Drawing for the job (mm, zero at the part's lowest x, y, z). A direction names the side the tool comes from. Give positions to 0.01 mm unless a question says otherwise; leave off trailing zeros. Order: outer loops, then holes, each group sorted by start corner. A loop starts at its lowest first (then second) coordinate and runs counter-clockwise, first axis right, second up. Notation, with made-up numbers: M 18.5,32 L 30.5,32 A12 ccw 30.5,45 Z; hole C 83.25,76 d1. An arc over 180 degrees is marked long. Answer as a JSON object with one key per item and string values.
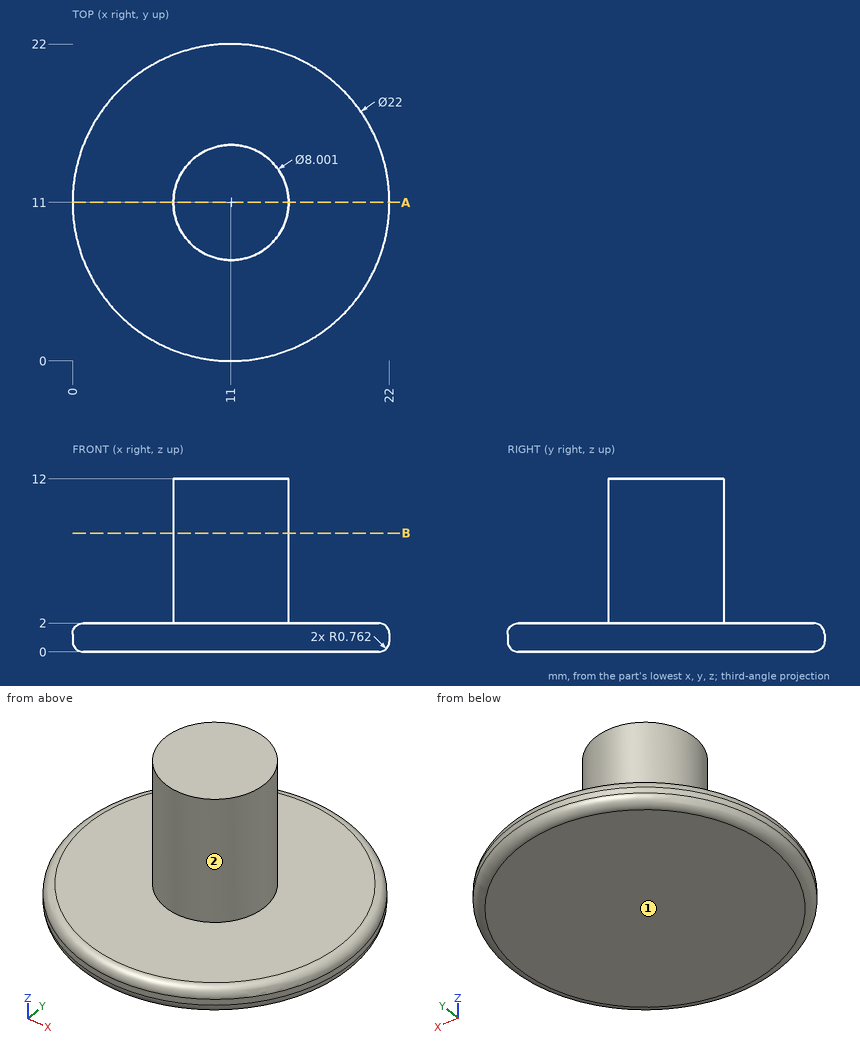
1. Cut at A-A on y = 11. Give the cut face in (x, z).
Worked answers:
{"outline": "M 0,0.76 A0.76 ccw 0.76,0 L 21.24,0 A0.76 ccw 22,0.76 L 22,1.24 A0.76 ccw 21.24,2 L 15,2 L 15,12 L 7,12 L 7,2 L 0.76,2 A0.76 ccw 0,1.24 Z"}
2. Pin check, flat tip, straight feed: P1, Ø5, axis at x = 6.5, y = 5.5, coming from the -Z side. Stop position of the tip, or through.
Worked answers:
{"P1": "stops at z = 0"}
3. Probe line 1 along Z through (x, y) = (18.5, 8); line 2 along Y through (x, z) = (17.25, 1.5); line 3 along Y through (x, z) = (20.25, 1.75). List the from-to ranges inside material, lowest first.
Worked answers:
{"line 1": "z = 0 to 2", "line 2": "y = 2 to 20", "line 3": "y = 5.42 to 16.58"}
4. Which spindle directions (+Z, -Z, +X, -X, +Y, -Y) get a long thin tool onto all of the face, cutting with end or side? Do the marked faces 1 and 2. Say none if no direction does.
Worked answers:
{"face 1": "-Z, +X, -X, +Y, -Y", "face 2": "+Z"}
5. Cut at B-B on z = 8.25. Give the cut face in (x, y).
Worked answers:
{"outline": "C 11,11 d8"}
